Autodesk Inventor part; units mm, degrees
ref_plane "YZ Plane" through (0, 0, 0) normal (1, 0, 0) x (0, 1, 0)
ref_plane "XZ Plane" through (0, 0, 0) normal (0, 1, 0) x (-1, 0, 0)
ref_plane "XY Plane" through (0, 0, 0) normal (0, 0, 1) x (1, 0, 0)
sketch "Sketch1" plane through (0, 0, 0) normal (0, 1, 0) x (-1, 0, 0)
  line L0 (15.1833, 0) -> (65, 0)
  line L1 (90, 0) -> (90, -18) construction
  line L2 (90, -90) -> (70, -90) construction
  line L3 (0, -90) -> (0, 0) construction
  line L4 (85, -18) -> (75, -18)
  line L5 (70, -18) -> (70, -72) construction
  line L6 (75, -72) -> (85, -72)
  line L7 (90, -67) -> (90, -18)
  circle A0 centre (80, -10) radius 10 construction
  circle A1 centre (80, -80) radius 10 construction
  circle A2 centre (80, -10) radius 1.25
  circle A3 centre (80, -80) radius 1.25
  circle A4 centre (60, -10) radius 1.25
  circle A5 centre (60, -80) radius 1.25
  circle A6 centre (40, -10) radius 1.25
  circle A7 centre (40, -80) radius 1.25
  circle A8 centre (20, -10) radius 1.25
  circle A9 centre (20, -80) radius 1.25
  circle A10 centre (0, -10) radius 1.25 construction
  circle A11 centre (0, -80) radius 1.25 construction
  line L8 (20, -10) -> (0, -80) construction
  circle A12 centre (10, -45) radius 7.9375
  circle A13 centre (10, -45) radius 20 construction
  line L9 (0, 0) -> (-10, 0) construction
  line L10 (-10, 0) -> (-10, -90) construction
  line L11 (-10, -90) -> (0, -90) construction
  circle A14 centre (1, -9) radius 3.5 construction
  circle A15 centre (1, -81) radius 3.5 construction
  line L12 (4.5, -90) -> (4.5, -81) construction
  line L13 (4.5, 0) -> (4.5, -9) construction
  line L14 (-8.44, -48.7987) -> (4.2376, -79.6704)
  line L15 (-8.44, -41.2013) -> (4.2376, -10.3296)
  line L16 (4.2376, -10.3296) -> (5.9329, -6.2013)
  line L17 (4.2376, -79.6704) -> (5.9329, -83.7987)
  arc A16 (15.1833, 0) -> (5.9329, -6.2013) centre (15.1833, -10) ccw
  arc A17 (5.9329, -83.7987) -> (15.1833, -90) centre (15.1833, -80) ccw
  arc A18 (-8.44, -41.2013) -> (-8.44, -48.7987) centre (0.8104, -45) ccw
  line L18 (90, -23) -> (90, -72)
  line L19 (90, -72) -> (90, -90) construction
  line L20 (70, -13) -> (70, -5)
  line L21 (70, -77) -> (70, -85)
  line L22 (65, -90) -> (15.1833, -90)
  arc A19 (70, -5) -> (65, 0) centre (65, -5) ccw
  arc A20 (70, -13) -> (75, -18) centre (75, -13) ccw
  arc A21 (90, -23) -> (85, -18) centre (85, -23) ccw
  arc A22 (85, -72) -> (90, -67) centre (85, -67) ccw
  arc A23 (75, -72) -> (70, -77) centre (75, -77) ccw
  arc A24 (65, -90) -> (70, -85) centre (65, -85) ccw
  line L23 (10, -45) -> (47.545, -45) construction
  circle A25 centre (47.545, -45) radius 7.9375
  point P0 (-10, -45)
  point P1 (8.4795, 0)
  point P2 (8.4795, -90)
  dimension "d0" = 90
  dimension "d1" = 90
  dimension "d2" = 20
  dimension "d3" = 54
  dimension "d4" = 18
  dimension "d5" = 2.5
  dimension "d8" = 70
  dimension "d11" = 20
  dimension "d14" = 15.875
  dimension "d15" = 40
  dimension "d17" = 7
  dimension "d18" = 89
  dimension "d19" = 7
  dimension "d20" = 0
  dimension "d21" = 72
  dimension "d22" = 9
  dimension "d23" = 10
  dimension "d24" = 10
  dimension "d25" = 5
  dimension "d26" = 37.545
  dimension "d27" = 15.875
extrude "Extrusion1" add sketch "Sketch1" along normal blind 3 contours L0 A19 L20 A20 L4 A21 L7 A22 L6 A23 L21 A24 L22 A17 L17 L14 A18 L15 L16 A16
equation "\"d4\" = -0.5 * d3 + 0.5 * d1"
equation "\"d22\" = -0.5 * d21 + 0.5 * d1"
equation "\"d27\" = d14"
properties part number "AntennaPlateUpper"
Here's how the part is built. I have some questions about the finished solid (model axes, mm). A direction names the side the tool comes from. Give positions to 0.01 mm unless a question says otherwise; leave off trailing zeros. Loops run counter-clockwise (first coordinate to the right, second up) from the corner with the lowest first, then second, coordinate; pieces in that order, holes last. Notation, with made-up numbers: M 27,36.5 L 49,36.5 A8 ccw 49,40.5 Z; hole C 46.5,80 d9. An arc over 180 degrees is marked long. Use one line per item in the form item = value. Start each with the question number.
Q1. Which directions (+Z, -Z, +X, -X, +Y, -Y) give clear straight access to the entire face, cutting with the end or side of a thin tool? Please do faces 1 (the flat face through (-80, 1, -18)), 2 (the cylindrical face through (-39.079, 1.479, -10.845)), 3 (the flat face through (-80, 1, -72)).
Q2. Will these pins go through, and if not, where does the flat tip stop? pin 1 Ø1.5 at (y, z) = (2, -8.5) entering from -X; pin 2 Ø1 at (y, z) = (1.5, -17) entering from +X.
Q3. Thinking about a two-plate mould opening in Z: for faces 4 (the cylindrical face through (-39.84, 1.48, -81.24)), 5 (the cylindrical face through (-61.19, 1.48, -10.38)), 6 (the flat face through (-90, 1, -45)), 7 (the flat face through (-40, 1, 0)), which applies, +Z half, -Z half, draft (parallel to the pull), parting line (faces both ways), or undercut?
Q4. If we section it at D-D (x = -8.5): Write out the boundary of the cut face in (y, z).
Q5. If we section it at B-B (z = -45): Write out the boundary of the cut face in (x, y).
Q6. If we section it at A-A (x = -60): Write out the boundary of the cut face in (y, z), then the cut area to 3 significant figures.
Q7. If we section it at C-C (y = 1.8): State how many separate pieces and enclosed holes the cut face has, then the cut area to 3 significant figures.
Q8. I need wall thicknesses on line 1 along Z through (x, y) = (-20, 1.5); line 2 along X through (y, z) = (1.25, -80); line 3 along X through (y, z) = (2.5, -39). Which ranges of each line are inside material? Lowest first, please.
Taken from the geometry:
q1.face_1 = +Z, -X, +Y, -Y
q1.face_2 = +Y, -Y
q1.face_3 = -Z, -X, +Y, -Y
q2.pin_1 = -70
q2.pin_2 = -1.29
q3.face_4 = undercut
q3.face_5 = undercut
q3.face_6 = draft
q3.face_7 = +Z half
q4.outline = M 0,-87.44 L 3,-87.44 L 3,-52.79 L 0,-52.79 Z; M 0,-37.21 L 3,-37.21 L 3,-2.56 L 0,-2.56 Z
q5.outline = M -90,0 L -55.48,0 L -55.48,3 L -90,3 Z; M -39.61,0 L -17.94,0 L -17.94,3 L -39.61,3 Z; M -2.06,0 L 9.19,0 L 9.19,3 L -2.06,3 Z
q6.outline = M 0,-90 L 3,-90 L 3,-81.25 L 0,-81.25 Z; M 0,-78.75 L 3,-78.75 L 3,-11.25 L 0,-11.25 Z; M 0,-8.75 L 3,-8.75 L 3,0 L 0,0 Z
q6.area = 255 mm^2
q7.separate_pieces = 1
q7.enclosed_holes = 8
q7.area = 6,990 mm^2
q8.line_1 = -90 to -81.25, -78.75 to -11.25, -8.75 to 0
q8.line_2 = -70 to -61.25, -58.75 to -41.25, -38.75 to -21.25, -18.75 to -4.37
q8.line_3 = -90 to -52.74, -42.35 to -15.2, -4.8 to 7.54
